Autodesk Inventor part; units mm, degrees
ref_plane "YZ Plane" through (0, 0, 0) normal (1, 0, 0) x (0, 1, 0)
ref_plane "XZ Plane" through (0, 0, 0) normal (0, 1, 0) x (-1, 0, 0)
ref_plane "XY Plane" through (0, 0, 0) normal (0, 0, 1) x (1, 0, 0)
sketch "Sketch1" plane through (0, 0, 0) normal (0, 1, 0) x (-1, 0, 0)
  line L0 (8.89, 0) -> (-8.89, 0) construction
  line L1 (8.89, 1.5875) -> (-8.89, 1.5875)
  line L2 (-8.89, -1.5875) -> (8.89, -1.5875)
  arc A0 (8.89, -1.5875) -> (8.89, 1.5875) centre (8.89, 0) ccw
  arc A1 (-8.89, 1.5875) -> (-8.89, -1.5875) centre (-8.89, 0) ccw
  line L3 (8.89, -5.0038) -> (-8.89, -5.0038) construction
  line L4 (8.89, -3.4163) -> (-8.89, -3.4163)
  line L5 (-8.89, -6.5913) -> (8.89, -6.5913)
  arc A2 (8.89, -6.5913) -> (8.89, -3.4163) centre (8.89, -5.0038) ccw
  arc A3 (-8.89, -3.4163) -> (-8.89, -6.5913) centre (-8.89, -5.0038) ccw
  line L6 (8.89, -10.0076) -> (-8.89, -10.0076) construction
  line L7 (8.89, -8.4201) -> (-8.89, -8.4201)
  line L8 (-8.89, -11.5951) -> (8.89, -11.5951)
  arc A4 (8.89, -11.5951) -> (8.89, -8.4201) centre (8.89, -10.0076) ccw
  arc A5 (-8.89, -8.4201) -> (-8.89, -11.5951) centre (-8.89, -10.0076) ccw
  line L9 (12.7, 20.1549) -> (-12.7, 20.1549)
  line L10 (-12.7, 20.1549) -> (-12.7, -17.9451)
  line L11 (-12.7, -17.9451) -> (12.7, -17.9451)
  line L12 (12.7, -17.9451) -> (12.7, 20.1549)
  line L13 (6.35, 13.8049) -> (-6.35, 13.8049) construction
  line L14 (-8.89, -16.5989) -> (8.89, -16.5989)
  arc A6 (8.89, -16.5989) -> (8.89, -13.4239) centre (8.89, -15.0114) ccw
  line L15 (8.89, -13.4239) -> (-8.89, -13.4239)
  line L16 (8.89, -15.0114) -> (-8.89, -15.0114) construction
  arc A7 (-8.89, -13.4239) -> (-8.89, -16.5989) centre (-8.89, -15.0114) ccw
  point P0 (0, 0)
  point P1 (0, -5.0038)
  point P2 (0, -10.0076)
  point P3 (10.4775, -5.0038)
  point P4 (10.4775, 0)
  point P5 (10.4775, -10.0076)
  point P6 (0, -17.9451)
  point P7 (0, -11.5951)
  point P8 (0, 13.8049)
  point P9 (0, 20.1549)
  point P10 (0, -16.5989)
  point P11 (10.4775, -15.0114)
  dimension "d1" = 17.78
  dimension "d3" = 3.175
  dimension "d4" = 5.0038
  dimension "d5" = 5.0038
  dimension "d8" = 25.4
  dimension "d9" = 38.1
  dimension "d10" = 6.35
  dimension "d11" = 12.7
  dimension "d12" = 6.35
  dimension "d25" = 5.0038
extrude "Extrusion1" add sketch "Sketch1" along normal blind 1.524
hole "Hole1" at (-6.35, 0, 13.8049) at (6.35, 0, 13.8049) direction (0, 1, 0) diameter 5.1054 end through all
fillet "Fillet1" radius 3.175 4 edges at (-12.7, 0.762, -17.9451) (12.7, 0.762, -17.9451) (12.7, 0.762, 20.1549) (-12.7, 0.762, 20.1549)
sketch "Sketch2" plane through (0, 1.524, 0) normal (0, 1, 0) x (1, 0, 0)
  line L0 (-12.7, 20.6375) -> (12.7, 20.6375)
  line L1 (12.7, 20.6375) -> (12.7, -4.7625)
  line L2 (12.7, -4.7625) -> (-12.7, -4.7625)
  line L3 (-12.7, -4.7625) -> (-12.7, 20.6375)
  line L4 (9.525, 17.9451) -> (-9.525, 17.9451) construction
  line L5 (8.89, -1.5875) -> (-8.89, -1.5875) construction
  point P0 (0, 0)
  point P1 (0, 20.6375)
  point P2 (0, 17.9451)
  dimension "d30" = 25.4
  dimension "d31" = 25.4
  dimension "d32" = 3.175
extrude "Extrusion2" cut sketch "Sketch2" against normal through all
fillet "Fillet2" radius 3.175 2 edges at (12.7, 0.762, 4.7625) (-12.7, 0.762, 4.7625)
properties part number "EL2-033" material "ABS Plastic"
Could you check a few things on this model? Use its own coordinates, in mm. Coordinates: 2 decimals unless noted, no trailing zeros. Loops run counter-clockwise (first coordinate to the right, second up) from the corner with the lowest first, then second, coordinate; pieces in that order, holes last.
1. We'd pull the mould along X, two halves only. Please class faces 1 (the face through (-4.797, 0.773, 15.831)), 2 (the face through (0, 1.524, 13)), 3 (the face through (12.7, 1, 13)), 4 (the face through (-11.795, 0.751, 5.717)): released by +X, released by -X, zero draft, split by the parting line, or undercut.
2. I need wall thicknesses on L1, parallel to Z at x = 6.35, y = 1.15; L2, parallel to X at y = 0.9, z = 13; L3, parallel to X at y = 1.25, z = 12.5. Which ranges of each line are inside material? Lowest first, please.
3. Imagine slicing it at A-A (x = -6.35). Please give me the cut outline in (y, z), and give its area (3 significant figures).
4. Imagine slicing it at C-C (z = 14.5). Please give me the cut outline in (x, y), and give its area (3 significant figures).
5. Imagine slicing it at B-B (y = 0.55). Give the number of separate pieces and of enclosed holes in the cut face, and give its area (3 significant figures).
6. Imagine slicing it at D-D (z = 19). Please give me the cut outline in (x, y).
Computed values:
1. face 1: undercut
1. face 2: zero draft
1. face 3: released by +X
1. face 4: released by -X
2. L1: z = 4.76 to 11.25, 16.36 to 20.15
2. L2: x = -12.7 to -8.77, -3.93 to 3.93, 8.77 to 12.7
2. L3: x = -12.7 to -8.54, -4.16 to 4.16, 8.54 to 12.7
3. outline: (0, 4.76) - (1.52, 4.76) - (1.52, 11.25) - (0, 11.25) - close; (0, 16.36) - (1.52, 16.36) - (1.52, 20.15) - (0, 20.15) - close
3. area: 15.7 mm2
4. outline: (-12.7, 0) - (-8.81, 0) - (-8.81, 1.52) - (-12.7, 1.52) - close; (-3.89, 0) - (3.89, 0) - (3.89, 1.52) - (-3.89, 1.52) - close; (8.81, 0) - (12.7, 0) - (12.7, 1.52) - (8.81, 1.52) - close
4. area: 23.7 mm2
5. separate pieces: 1
5. enclosed holes: 2
5. area: 341 mm2
6. outline: (-11.97, 0) - (11.97, 0) - (11.97, 1.52) - (-11.97, 1.52) - close
